The listing builds one solid part. Answer for the finished solid, in the listing's coordinates (mm). A direction names the side the tool comes from. Coordinates: 2 decimals unless noted, no trailing zeros. Order: outer loops, then holes, each group sorted by start corner. A loop starts at its lowest first (then second) coordinate and runs counter-clockwise, first axis right, second up. Notation, with made-up numbers: (67.5, 51) -> (119.5, 51) arc R33 cw to (119.5, 84) -> close; hole circle Ø8 at (41.5, 1.5). An arc over 180 degrees is marked (long way). Write each question's results on one line, items separated by ' | '. Start each with the question number.
(1) The part is cut by section D-D, the plane z = 4.5. Give the vertices of the cut face in (x, y), then the cut area to 3 significant figures.
(2) The part is cut by section A-A, the plane x = 0. Give the vertices of the cut face in (y, z), then the cut area to 3 significant figures.
(3) A tool of negligible diameter and unlimited length cuts with its end or side. For faces 4 (the face through (-0.1, 1, 26.9)), 5 (the face through (0.1, 1, 17.4)), 6 (the face through (-2.75, 1, 22)), from which of +Z, -Z, +X, -X, +Y, -Y can it reach the whole face along a straight path? Write none if from no direction.
(4) The part is cut by section B-B, the plane z = 0. Give the vertices of the cut face in (x, y), then the cut area to 3 significant figures.
(5) Straight lines are drawn through the part: L1, parallel to X at y = 2.8, z = 20; L2, parallel to X at y = 3.1, z = 24.15; L3, parallel to Z at x = -1.5, y = 2.65. For each, find the intervals that lie inside material, in ascending order.
(6) Given pin 1 (2 mm diameter, centred on y = 5, z = 15.5, fed in from -X); pin 2 (3 mm diameter, centred on x = 0, z = 24.15, fed in from -Y); pin 3 (2 mm diameter, centred on y = 1.5, z = 21.5, fed in from +X); pin 4 (1 mm diameter, centred on y = 1, z = 22.5, fed in from -X), each flat-ended and moving along its own axis, determine where each tip first touches the part or whether it passes through.
(7) The part is cut by section C-C, the plane z = 20.5. Give the vertices of the cut face in (x, y), then the cut area to 3 significant figures.
(8) Determine the mould class of faces 1 (the face through (-3.35, 4, 17)), 2 (the face through (0.9, 2.96, 2.86)), 3 (the face through (-3.796, 4.028, 7.238)) for opening direction Z: +Z half, -Z half, draft (parallel to the pull), parting line (faces both ways), or undercut.
```python
from build123d import *
from build123d.topology import SkipClean

# Parameters (mm, degrees)
ESQUISSE1_R             = 3
BOSS_EXTRU_1_DEPTH      = 6
D_GAGEMENT_M31_D        = 3.4
ENL_V_MAT_EXTRU_1_DEPTH = 2
CONG_2_R                = 5


with BuildPart() as part:
    # Esquisse1 → Boss.-Extru.1 (new body)
    with BuildSketch(Plane(origin=(0, 0, 0), x_dir=(1, 0, 0), z_dir=(0, 1, 0))):
        with BuildLine():
            Line((-3.35, -24.15), (-3.35, -6.710253348))
            ThreePointArc((-3.35, -6.710253348), (0, 7.5), (3.35, -6.710253348))
            Line((3.35, -6.710253348), (3.35, -24.15))
            ThreePointArc((3.35, -24.15), (0, -27.5), (-3.35, -24.15))
        make_face()
        with Locations(Location((0, 0, 0), (0, 0, 270))):
            Circle(ESQUISSE1_R, mode=Mode.SUBTRACT)
    extrude(amount=BOSS_EXTRU_1_DEPTH)

    # Dégagement M31 (through all)
    with Locations(Plane(origin=(0, 0, 0), x_dir=(-1, 0, 0), z_dir=(0, -1, 0))):
        with Locations((0, -24.15), (0, -20.15)):
            Hole(D_GAGEMENT_M31_D / 2)

    # Esquisse6 → Enlèv. mat.-Extru.1 (cut)
    with SkipClean():  # the faces are left unmerged after this step: merging them gives an invalid solid
        with BuildSketch(Plane.XZ):
            with BuildLine():
                Line((-3.35, 24.15), (-3.35, 6.710253348))
                ThreePointArc((-3.35, 6.710253348), (0, 7.5), (3.35, 6.710253348))
                Line((3.35, 6.710253348), (3.35, 24.15))
                ThreePointArc((3.35, 24.15), (0, 27.5), (-3.35, 24.15))
            make_face()
            with BuildLine():
                Line((2.75, 24.15), (2.75, 20.15))
                ThreePointArc((2.75, 20.15), (0, 17.4), (-2.75, 20.15))
                Line((-2.75, 20.15), (-2.75, 24.15))
                ThreePointArc((-2.75, 24.15), (0, 26.9), (2.75, 24.15))
            make_face(mode=Mode.SUBTRACT)
        extrude(amount=-ENL_V_MAT_EXTRU_1_DEPTH, mode=Mode.SUBTRACT)

    # Congé2
    cong_2_edges = [part.edges().sort_by_distance(p)[0] for p in [
        (-3.35, 4, 6.710253348),
        (3.35, 4, 6.710253348),
    ]]
    fillet(cong_2_edges, radius=CONG_2_R)


solid = part.part
```
Established:
1) outline: (-6, 0) -> (6, 0) -> (6, 6) -> (-6, 6) -> close | area: 72.0 mm^2
2) outline: (0, -7.5) -> (6, -7.5) -> (6, -3) -> (0, -3) -> close; (0, 3) -> (6, 3) -> (6, 18.45) -> (0, 18.45) -> (0, 17.4) -> (2, 17.4) -> (2, 7.5) -> (0, 7.5) -> close; (0, 21.85) -> (6, 21.85) -> (6, 22.45) -> (0, 22.45) -> close; (0, 25.85) -> (6, 25.85) -> (6, 27.5) -> (2, 27.5) -> (2, 26.9) -> (0, 26.9) -> close | area: 112 mm^2
3) face 4: +Z, -Y | face 5: -Y | face 6: +Z, -X, -Y
4) outline: (-7.5, 0) -> (-3, 0) -> (-3, 6) -> (-7.5, 6) -> close; (3, 0) -> (7.5, 0) -> (7.5, 6) -> (3, 6) -> close | area: 54.0 mm^2
5) L1: x = -3.35 to -1.69, 1.69 to 3.35 | L2: x = -3.35 to -1.7, 1.7 to 3.35 | L3: z = -7.35 to -2.6, 2.6 to 19.35, 20.95 to 23.35, 24.95 to 27.15
6) pin 1: stops at x = -3.35 | pin 2: passes through | pin 3: stops at x = 3.35 | pin 4: stops at x = -2.75
7) outline: (-3.35, 2) -> (-2.75, 2) -> (-2.75, 0) -> (-1.66, 0) -> (-1.66, 6) -> (-3.35, 6) -> close; (1.66, 0) -> (2.75, 0) -> (2.75, 2) -> (3.35, 2) -> (3.35, 6) -> (1.66, 6) -> close | area: 17.8 mm^2
8) face 1: draft | face 2: undercut | face 3: +Z half
